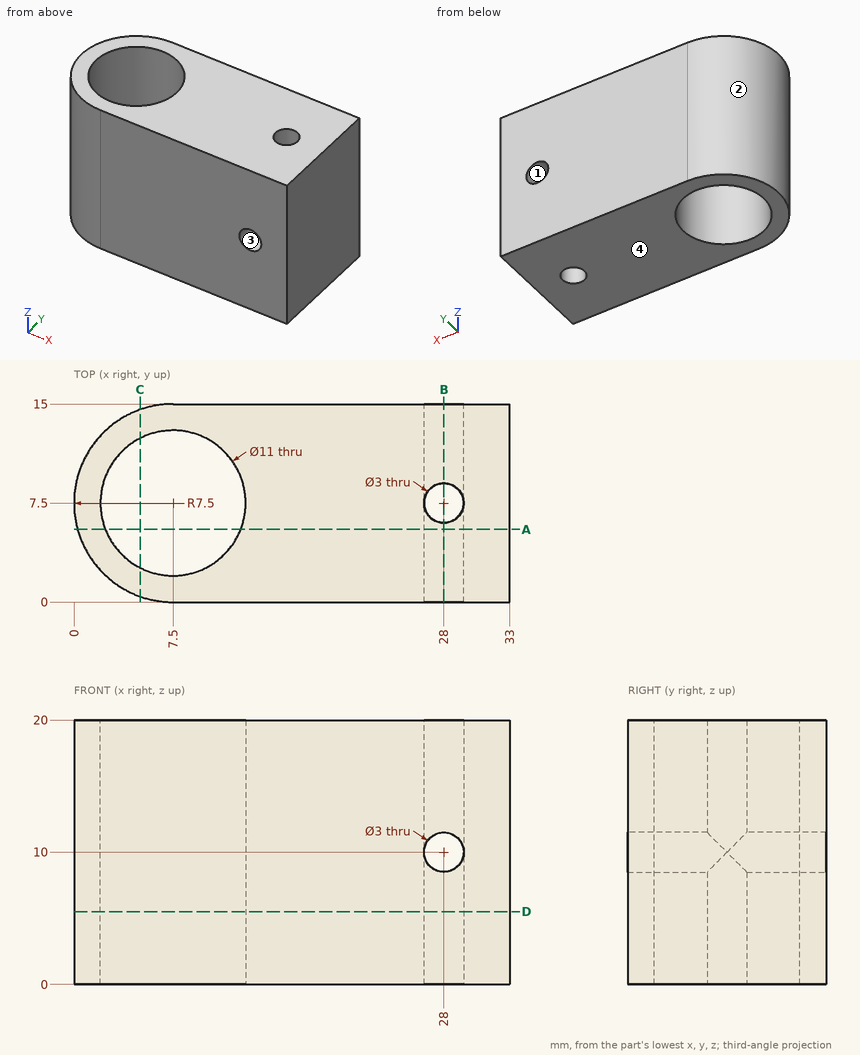
Answer from the drawing. Dimensions are ordinates in mm from the lowest x, y and z of the part. Give positions to 0.01 mm unless a question says otherwise; leave off trailing zeros. Order: outer loops, then holes, each group sorted by start corner. A loop starts at its lowest first (then second) coordinate and runs counter-clockwise, first axis right, second up. Notation, with made-up numbers: (-7, 47.25) - (48, 47.25) arc R21 ccw to (48, 86.25) - close; hole circle Ø5 at (77, -22.75). An arc over 180 degrees is marked (long way). One line per item, written item: value. Start each with the question number.
1. For a pull along Z with two mould halves and no side action, classify the marked faces 1, 2, 3 and 4 as released by +Z, released by -Z, zero draft, split by the parting line, or undercut.
2. Each of these flat-tipped pins is pushed along its axis until it touches: pin 1 Ø3.5 at (x, z) = (28, 10) entering from -Y; pin 2 Ø1 at (y, z) = (5, 14) entering from -X; pin 3 Ø1.5 at (x, z) = (4.5, 12) entering from -Y. Where does it stop, or does it pass through?
3. Section B-B, the plane x = 28 is taken. Write down the section's boundary in (y, z), then the cut area to 3 significant figures.
4. Section C-C, the plane x = 5 is taken. Write down the section's boundary in (y, z).
5. Section A-A, the plane y = 5.5 is taken. Write down the section's boundary in (x, z), then the cut area to 3 significant figures.
6. Section D-D, the plane z = 5.5 is taken. Write down the section's boundary in (x, y).
7. Consider line 1 (X direction, y = 4, z = 10); line 2 (X direction, y = 5.25, z = 10); line 3 (Z direction, x = 28, y = 3.25). Determine where each line is inside the solid, lowest interval first.
Filled sheet:
1. face 1: undercut
1. face 2: zero draft
1. face 3: undercut
1. face 4: released by -Z
2. pin 1: y = 0
2. pin 2: x = 0.27
2. pin 3: y = 0.35
3. outline: (0, 0) - (6, 0) - (6, 8.5) - (0, 8.5) - close; (0, 11.5) - (6, 11.5) - (6, 20) - (0, 20) - close; (9, 0) - (15, 0) - (15, 8.5) - (9, 8.5) - close; (9, 11.5) - (15, 11.5) - (15, 20) - (9, 20) - close
3. area: 204 mm²
4. outline: (0.43, 0) - (2.6, 0) - (2.6, 20) - (0.43, 20) - close; (12.4, 0) - (14.57, 0) - (14.57, 20) - (12.4, 20) - close
5. outline: (0.27, 0) - (2.38, 0) - (2.38, 20) - (0.27, 20) - close; (12.62, 0) - (33, 0) - (33, 20) - (12.62, 20) - close; hole circle Ø3 at (28, 10)
5. area: 443 mm²
6. outline: (7.5, 0) - (33, 0) - (33, 15) - (7.5, 15) arc R7.5 ccw to start; hole circle Ø11 at (7.5, 7.5); hole circle Ø3 at (28, 7.5)
7. line 1: 0.87 to 3.26, 11.74 to 26.5, 29.5 to 33
7. line 2: 0.35 to 2.48, 12.52 to 26.5, 29.5 to 33
7. line 3: 0 to 8.5, 11.5 to 20
